The listing builds one solid part. Answer for the finished solid, in the listing's coordinates (mm). A direction names the side the tool comes from. Round coordinates to 2 decimals unless told otherwise and drop trailing zeros. Loops run counter-clockwise (first coordinate to the right, second up) from the corner with the lowest first, then second, coordinate; pieces in that order, holes last. Notation, with made-up numbers: (54, -25.75) -> (73, -25.75) arc R28 cw to (73, 9.25) -> close; hole circle Ø5 at (60.5, 56.5). An arc over 180 degrees is marked (long way). Write each question's results on one line, items separated by ' | '. Start each with the question number.
(1) Determine the mould class of faces 1 (the face through (10, 2, -1)), 2 (the face through (0, 44.3, 62)), 3 (the face through (-54.95, 22.33, 2.35)) for opening direction Z: released by +Z, released by -Z, zero draft, split by the parting line, or undercut.
(2) Flat-ended cylindrical pins translate along their axes: pin 1 (1 mm diameter, centred on x = -18.5, z = -31.5, fed in from -Y); pin 2 (5 mm diameter, centred on y = 37.5, z = 28.5, fed in from +X); pin 3 (8 mm diameter, centred on y = 32.5, z = 19.5, fed in from +X); pin 4 (2.5 mm diameter, centred on x = -29.44, z = -35.34, fed in from -Y) (3 decimals). Find the tip coordinate at first contact, or state that the pin passes through.
(3) For faces 4 (the face through (46, 45.3, 23)), 5 (the face through (30.119, 2.493, 33.196)), 6 (the face through (-15.02, 1.01, 47.69)), 7 (the face through (15.02, 24.45, 47.69)), 8 (the face through (62, 44.3, 0)), determine the directions among +Z, -Z, +X, -X, +Y, -Y from which every point of the face is accessible in a straight line to the end or side of a thin tool.
(4) Straight lines are drawn through the part: probe 1 along X at (y, z) = (44.75, 0); probe 2 along X at (y, z) = (23, 0); probe 3 along Y at (x, z) = (37, -22). For each, find the intervals that lie inside material, in ascending order.
(5) The part is cut by section B-B (x = 0). Determine the outline of the cut face in (y, z).
(6) The part is cut by section D-D (z = 14). Determine the outline of the cut face in (x, y), plus the area to 3 significant figures.
(7) The part is cut by section A-A (z = 0). Determine the outline of the cut face in (x, y).
(8) The part is cut by section C-C (y = 13). Determine the outline of the cut face in (x, z), plus the area to 3 significant figures.
```python
from build123d import *

# Parameters (mm, degrees)
EXTRUDE_1_DEPTH     = 45.3
SKETCH_2_R          = 50
CUT_EXTRUDE_1_DEPTH = 42.3
CUT_EXTRUDE_3_DEPTH = 44.3
CUT_EXTRUDE_START   = -2
SKETCH_5_R          = 50
CUT_EXTRUDE_4_DEPTH = 2
SKETCH_6_R          = 2.25
CUT_EXTRUDE_5_DEPTH = 101.777676099
SKETCH_7_R          = 2.5
CUT_EXTRUDE_6_DEPTH = 101.777676099
SKETCH_8_R          = 2.5
CUT_EXTRUDE_7_DEPTH = 102.211362998
EXTRUDE_2_DEPTH     = 1
SKETCH_10_R         = 2.5
CUT_EXTRUDE_8_DEPTH = 1


with BuildPart() as part:
    # 草图1 → 凸台-拉伸1 (new body)
    with BuildSketch(Plane(origin=(0, 0, 0), x_dir=(1, 0, 0), z_dir=(0, 1, 0))):
        with BuildLine():
            Line((54.772255751, 5), (67.5, 5))
            ThreePointArc((67.5, 5), (72.5, 0), (67.5, -5))
            Line((67.5, -5), (54.772255751, -5))
            ThreePointArc((54.772255751, -5), (-55, 0), (54.772255751, 5))
        make_face()
    extrude(amount=EXTRUDE_1_DEPTH)

    # 草图2 → 切除-拉伸1 (cut)
    with BuildSketch(Plane(origin=(0, 45.3, 0), x_dir=(1, 0, 0), z_dir=(0, 1, 0))):
        with Locations(Location((0, 0, 0), (0, 0, 270))):
            Circle(SKETCH_2_R)
    extrude(amount=-CUT_EXTRUDE_1_DEPTH, mode=Mode.SUBTRACT)

    # 草图4 → 切除-拉伸3 (cut)
    with BuildSketch(Plane.XZ):
        with BuildLine():
            Line((67.5, 5), (67.5, -5))
            ThreePointArc((67.5, -5), (72.5, 0), (67.5, 5))
        make_face()
        with BuildLine():
            ThreePointArc((72.5, 0), (71.035533906, 3.535533906), (67.5, 5))
            Line((67.5, 5), (67.5, -5))
            ThreePointArc((67.5, -5), (71.035533906, -3.535533906), (72.5, 0))
        make_face()
        with BuildLine():
            Line((67.5, -5), (67.5, 5))
            ThreePointArc((67.5, 5), (62.5, 0), (67.5, -5))
        make_face()
        with BuildLine():
            Line((67.5, 5), (54.772255751, 5))
            Line((54.772255751, 5), (54.772255751, -5))
            Line((54.772255751, -5), (67.5, -5))
            ThreePointArc((67.5, -5), (62.5, 0), (67.5, 5))
        make_face()
    extrude(amount=-CUT_EXTRUDE_3_DEPTH, mode=Mode.SUBTRACT)

    # 草图5 → 切除-拉伸4 (cut)
    with BuildSketch(Plane.XZ.offset(CUT_EXTRUDE_START)):
        with Locations(Location((0, 0, 0), (0, 0, 90))):
            Circle(SKETCH_5_R)
    extrude(amount=CUT_EXTRUDE_4_DEPTH, mode=Mode.SUBTRACT)

    # 草图6 → 切除-拉伸5 (cut, through all)
    with BuildSketch(Plane(origin=(0, 2, 0), x_dir=(-1, 0, 0), z_dir=(0, -1, 0))):
        with Locations(Location((-4.170920038, 45.810516544, 0), (0, 0, 90))):
            Circle(SKETCH_6_R)
        with Locations(Location((29.443641055, 35.342212741, 0), (0, 0, 90))):
            Circle(SKETCH_6_R)
        with Locations(Location((45.810516544, 4.170920038, 0), (0, 0, 90))):
            Circle(SKETCH_6_R)
        with Locations(Location((35.342212741, -29.443641055, 0), (0, 0, 90))):
            Circle(SKETCH_6_R)
        with Locations(Location((4.170920038, -45.810516544, 0), (0, 0, 90))):
            Circle(SKETCH_6_R)
        with Locations(Location((-29.443641055, -35.342212741, 0), (0, 0, 90))):
            Circle(SKETCH_6_R)
        with Locations(Location((-45.810516544, -4.170920038, 0), (0, 0, 90))):
            Circle(SKETCH_6_R)
        with Locations(Location((-35.342212741, 29.443641055, 0), (0, 0, 90))):
            Circle(SKETCH_6_R)
    extrude(amount=-CUT_EXTRUDE_5_DEPTH, mode=Mode.SUBTRACT)

    # 草图7 → 切除-拉伸6 (cut, through all)
    with BuildSketch(Plane.XZ.offset(-2)):
        with Locations(Location((0, 0, 0), (0, 0, 270))):
            Circle(SKETCH_7_R)
    extrude(amount=-CUT_EXTRUDE_6_DEPTH, mode=Mode.SUBTRACT)

    # 草图8 → 切除-拉伸7 (cut, through all)
    with BuildSketch(Plane.XZ.offset(-44.3)):
        with Locations(Location((67.5, 0, 0), (0, 0, 270))):
            Circle(SKETCH_8_R)
    extrude(amount=-CUT_EXTRUDE_7_DEPTH, mode=Mode.SUBTRACT)

    # 草图9 → 凸台-拉伸2 (add)
    with BuildSketch(Plane(origin=(0, 45.3, 0), x_dir=(1, 0, 0), z_dir=(0, 1, 0))):
        with BuildLine():
            Line((5, -67.5), (5, -54.718723613))
            Line((5, -54.718723613), (0, -55))
            Line((0, -55), (-5, -54.718723613))
            Line((-5, -54.718723613), (-5, -67.5))
            ThreePointArc((-5, -67.5), (0, -72.5), (5, -67.5))
        make_face()
    extrude(amount=-EXTRUDE_2_DEPTH)

    # 草图10 → 切除-拉伸8 (cut)
    with BuildSketch(Plane(origin=(0, 45.3, 0), x_dir=(1, 0, 0), z_dir=(0, 1, 0))):
        with Locations(Location((0, -67.5, 0), (0, 0, 270))):
            Circle(SKETCH_10_R)
    extrude(amount=-CUT_EXTRUDE_8_DEPTH, mode=Mode.SUBTRACT)


solid = part.part
```
Checked values:
1) face 1: undercut | face 2: zero draft | face 3: split by the parting line
2) pin 1: stops at y = 2 | pin 2: stops at x = 48.47 | pin 3: stops at x = 52.77 | pin 4: passes through
3) face 4: +Z, -Z, +X, -X, +Y | face 5: +Y, -Y | face 6: -Y | face 7: +Y | face 8: +Z, -Z, +X, -Y
4) probe 1: x = -55 to -50, 50 to 65, 70 to 72.5 | probe 2: x = -55 to -50, 50 to 54.77 | probe 3: y = 2 to 3
5) outline: (0, -55) -> (45.3, -55) -> (45.3, -50) -> (3, -50) -> (3, -2.5) -> (2, -2.5) -> (2, -50) -> (0, -50) -> close; (0, 50) -> (2, 50) -> (2, 2.5) -> (3, 2.5) -> (3, 50) -> (45.3, 50) -> (45.3, 65) -> (44.3, 65) -> (44.3, 55) -> (0, 55) -> close; (44.3, 70) -> (45.3, 70) -> (45.3, 72.5) -> (44.3, 72.5) -> close
6) outline: (-53.19, 0) -> (-48, 0) -> (-48, 2) -> (48, 2) -> (48, 0) -> (53.19, 0) -> (53.19, 45.3) -> (48, 45.3) -> (48, 3) -> (-48, 3) -> (-48, 45.3) -> (-53.19, 45.3) -> close | area: 566 mm2
7) outline: (-55, 0) -> (-50, 0) -> (-50, 2) -> (-2.5, 2) -> (-2.5, 3) -> (-50, 3) -> (-50, 45.3) -> (-55, 45.3) -> close; (2.5, 2) -> (50, 2) -> (50, 0) -> (54.77, 0) -> (54.77, 44.3) -> (65, 44.3) -> (65, 45.3) -> (50, 45.3) -> (50, 3) -> (2.5, 3) -> close; (70, 44.3) -> (72.5, 44.3) -> (72.5, 45.3) -> (70, 45.3) -> close
8) outline: (54.77, -5) -> (54.77, 5) arc R55 ccw (long way) to start; hole circle Ø100 at (0, 0) | area: 1,650 mm2
